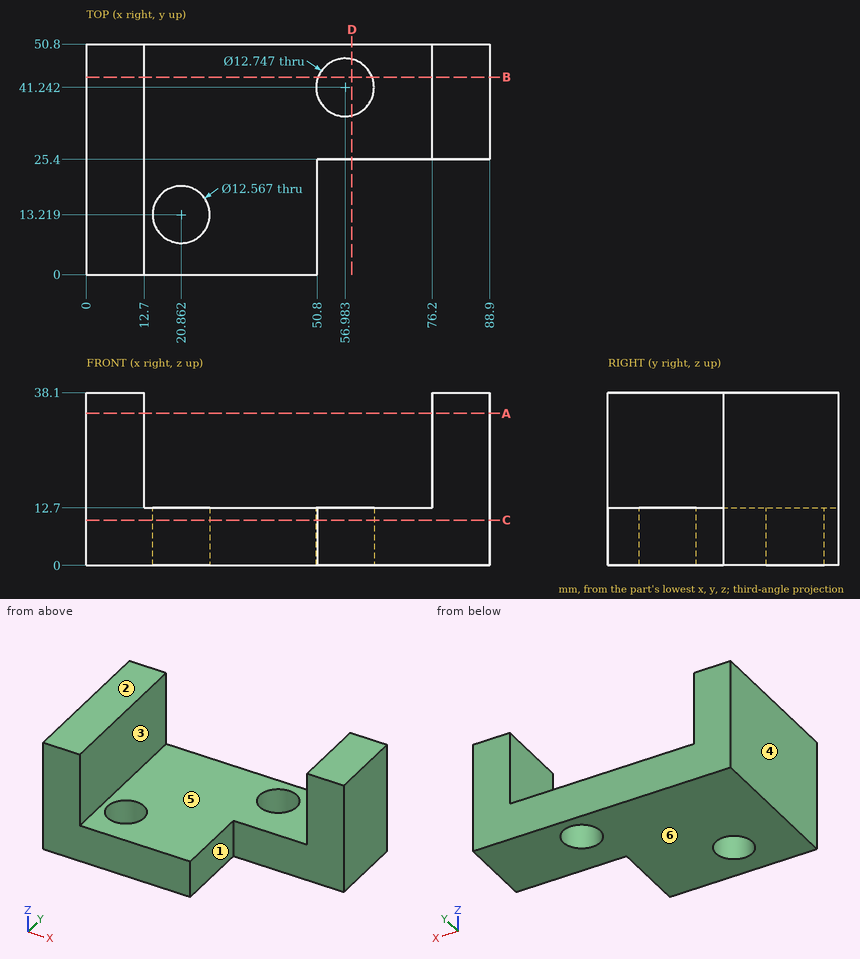
Job drawing, mm, ordinate dimensions from the low corner. One solid piece. A direction names the side the tool comes from. Round coordinates to 2 decimals unless told otherwise and drop trailing zeros. Order: outer loops, then holes, each group sorted by start corner. A loop starts at its lowest first (then second) coordinate and runs counter-clockwise, first axis right, second up. Notation, with made-up numbers: (20, 5.5) -> (48, 5.5) arc R21 ccw to (48, 41.5) -> close; hole circle Ø6 at (46, 9). An arc over 180 degrees is marked (long way). Answer in a Markdown table with one row per item.
1) Band-saw the part on B-B on y = 43.5. Give the cut face in (x, z).
Values:
| item | result |
|---|---|
| outline | (0, 0) -> (51.02, 0) -> (51.02, 12.7) -> (12.7, 12.7) -> (12.7, 38.1) -> (0, 38.1) -> close; (62.94, 0) -> (88.9, 0) -> (88.9, 38.1) -> (76.2, 38.1) -> (76.2, 12.7) -> (62.94, 12.7) -> close |
2) Which spindle directions (+Z, -Z, +X, -X, +Y, -Y) get a long thin tool onto all of the face, cutting with end or side? Do the marked faces 1, 2 and 3. Say none if no direction does.
Values:
| item | result |
|---|---|
| face 1 | +Z, -Z, +X, -Y |
| face 2 | +Z, +X, -X, +Y, -Y |
| face 3 | +Z, +Y, -Y |
3) Wall check: L1, parallel to X at y = 44, z = 25.5; L2, parallel to X at y = 20.5, z = 5; L3, parallel to Z at x = 42.5, y = 24.5. Give the ranges that are in metal, low to high.
Values:
| item | result |
|---|---|
| L1 | 0 to 12.7, 76.2 to 88.9 |
| L2 | 0 to 50.8 |
| L3 | 0 to 12.7 |
4) Band-saw the part on C-C on z = 10. Give the cut face in (x, y) (1 decimal).
Values:
| item | result |
|---|---|
| outline | (0, 0) -> (50.8, 0) -> (50.8, 25.4) -> (88.9, 25.4) -> (88.9, 50.8) -> (0, 50.8) -> close; hole circle Ø12.6 at (20.9, 13.2); hole circle Ø12.7 at (57, 41.2) |
5) Band-saw the part on D-D on x = 58.5. Give the cut face in (y, z), and give its area (3 significant figures).
Values:
| item | result |
|---|---|
| outline | (25.4, 0) -> (35.05, 0) -> (35.05, 12.7) -> (25.4, 12.7) -> close; (47.43, 0) -> (50.8, 0) -> (50.8, 12.7) -> (47.43, 12.7) -> close |
| area | 165 mm2 |
6) Band-saw the part on A-A on z = 33.5. Give the cut face in (x, y).
Values:
| item | result |
|---|---|
| outline | (0, 0) -> (12.7, 0) -> (12.7, 50.8) -> (0, 50.8) -> close; (76.2, 25.4) -> (88.9, 25.4) -> (88.9, 50.8) -> (76.2, 50.8) -> close |
7) Pin check, flat tips, straight feed: P1, Ø14, axis at y = 15.5, z = 9.5, coming from the +X side; P2, Ø16.5, axis at x = 20.86, y = 13.22, coming from the +Z side; P3, Ø5, axis at x = 44, z = 17.5, coming from the -Y side; P4, Ø20.5, axis at x = 56.98, y = 41.24, coming from the +Z side. Stop position of each tip, or through.
Values:
| item | result |
|---|---|
| P1 | x = 50.8 |
| P2 | z = 38.1 |
| P3 | through |
| P4 | z = 12.7 |
8) Mould opens along X. For the marked faces 4, 5 and 6 say: released by +X, released by -X, zero draft, split by the parting line, or undercut.
Values:
| item | result |
|---|---|
| face 4 | released by -X |
| face 5 | undercut |
| face 6 | zero draft |
